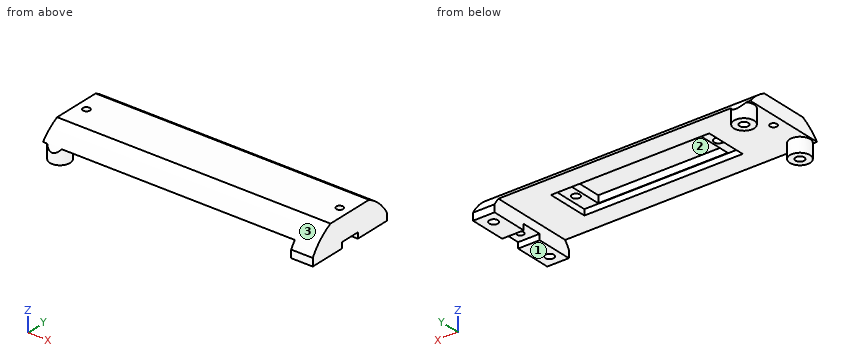
from build123d import *

# Parameters (mm, degrees)
SKETCH1_R             = 4
SKETCH1_R_2           = 1.5
BOSS_EXTRUDE1_DEPTH   = 5
BOSS_EXTRUDE1_2_DEPTH = 5
BOSS_EXTRUDE1_3_DEPTH = 5
BOSS_EXTRUDE1_4_DEPTH = 5
SKETCH2_W             = 95
SKETCH2_H             = 32.5
BOSS_EXTRUDE2_DEPTH   = 10
SKETCH3_W             = 45
SKETCH3_H             = 14.2
CUT_EXTRUDE1_DEPTH    = 9
SKETCH4_W             = 5
SKETCH4_H             = 14.2
SKETCH4_W_2           = 45
CUT_EXTRUDE2_DEPTH    = 4
SKETCH5_R             = 1.4
SKETCH5_R_2           = 1.6
CUT_EXTRUDE3_DEPTH    = 5
BOSS_EXTRUDE3_DEPTH   = 5
CUT_EXTRUDE5_DEPTH    = 96
SKETCH9_W             = 7
SKETCH9_H             = 7
CUT_EXTRUDE6_DEPTH    = 96
SKETCH10_R            = 1.2
CUT_EXTRUDE7_DEPTH    = 16
SKETCH12_R            = 1.5
CUT_EXTRUDE9_DEPTH    = 10
SKETCH13_W            = 95
SKETCH13_H            = 32.5
CUT_EXTRUDE10_DEPTH   = 5
SKETCH14_R            = 3.5
CUT_EXTRUDE11_DEPTH   = 5
SKETCH15_W            = 45
SKETCH15_H            = 14.2
CUT_EXTRUDE12_DEPTH   = 0.5
SKETCH16_R            = 1.4
SKETCH16_R_2          = 1.6
SKETCH16_W            = 45
SKETCH16_H            = 14.2
CUT_EXTRUDE13_DEPTH   = 2


with BuildPart() as part:
    # Sketch1 → Boss-Extrude1 (new body)
    with BuildSketch(Plane.XY):
        with Locations((-43.5, -12.25)):
            Circle(SKETCH1_R)
        with Locations((-43.5, -12.25)):
            Circle(SKETCH1_R_2, mode=Mode.SUBTRACT)
    extrude(amount=BOSS_EXTRUDE1_DEPTH)



with BuildPart() as body_2:
    # Sketch1 → Boss-Extrude1 2 (new body)
    with BuildSketch(Plane.XY):
        with Locations((-43.5, 12.25)):
            Circle(SKETCH1_R)
        with Locations((-43.5, 12.25)):
            Circle(SKETCH1_R_2, mode=Mode.SUBTRACT)
    extrude(amount=BOSS_EXTRUDE1_2_DEPTH)


with BuildPart() as body_3:
    # Sketch1 → Boss-Extrude1 3 (new body)
    with BuildSketch(Plane.XY):
        with Locations((43.5, -12.25)):
            Circle(SKETCH1_R)
        with Locations((43.5, -12.25)):
            Circle(SKETCH1_R_2, mode=Mode.SUBTRACT)
    extrude(amount=BOSS_EXTRUDE1_3_DEPTH)


with BuildPart() as body_4:
    # Sketch1 → Boss-Extrude1 4 (new body)
    with BuildSketch(Plane.XY):
        with Locations((43.5, 12.25)):
            Circle(SKETCH1_R)
        with Locations((43.5, 12.25)):
            Circle(SKETCH1_R_2, mode=Mode.SUBTRACT)
    extrude(amount=BOSS_EXTRUDE1_4_DEPTH)


with BuildPart() as part_1:
    add(part.part)

    add(body_2.part)  # Boss-Extrude2 merges body 2

    add(body_3.part)  # Boss-Extrude2 merges body 3

    add(body_4.part)  # Boss-Extrude2 merges body 4
    # Sketch2 → Boss-Extrude2 (add)
    with BuildSketch(Plane.XY.offset(5)):
        Rectangle(SKETCH2_W, SKETCH2_H)
    extrude(amount=BOSS_EXTRUDE2_DEPTH)

    # Sketch3 → Cut-Extrude1 (cut)
    with BuildSketch(Plane(origin=(0, 0, 5), x_dir=(-1, 0, 0), z_dir=(0, 0, -1))):
        Rectangle(SKETCH3_W, SKETCH3_H)
    extrude(amount=-CUT_EXTRUDE1_DEPTH, mode=Mode.SUBTRACT)

    # Sketch4 → Cut-Extrude2 (cut)
    with BuildSketch(Plane(origin=(0, 0, 5), x_dir=(-1, 0, 0), z_dir=(0, 0, -1))):
        with Locations((-25, 0)):
            Rectangle(SKETCH4_W, SKETCH4_H)
        Rectangle(SKETCH4_W_2, SKETCH4_H)
        with Locations((25, 0)):
            Rectangle(SKETCH4_W, SKETCH4_H)
    extrude(amount=-CUT_EXTRUDE2_DEPTH, mode=Mode.SUBTRACT)

    # Sketch5 → Cut-Extrude3 (cut)
    with BuildSketch(Plane(origin=(0, 0, 9), x_dir=(-1, 0, 0), z_dir=(0, 0, -1))):
        with Locations((-24.8, -0.2)):
            Circle(SKETCH5_R)
        with Locations((24.8, -0.2)):
            Circle(SKETCH5_R_2)
    extrude(amount=-CUT_EXTRUDE3_DEPTH, mode=Mode.SUBTRACT)

    # Sketch6 → Boss-Extrude3 (add)
    with BuildSketch(Plane(origin=(0, 0, 5), x_dir=(-1, 0, 0), z_dir=(0, 0, -1))):
        with BuildLine():
            ThreePointArc((47.5, 12.25), (43.5, 8.25), (39.5, 12.25))
            Line((39.5, 12.25), (39.5, -12.25))
            ThreePointArc((39.5, -12.25), (43.5, -8.25), (47.5, -12.25))
            Line((47.5, -12.25), (47.5, 12.25))
        make_face()
        with BuildLine():
            ThreePointArc((-39.5, 12.25), (-43.5, 8.25), (-47.5, 12.25))
            Line((-47.5, 12.25), (-47.5, -12.25))
            ThreePointArc((-47.5, -12.25), (-43.5, -8.25), (-39.5, -12.25))
            Line((-39.5, -12.25), (-39.5, 12.25))
        make_face()
    extrude(amount=BOSS_EXTRUDE3_DEPTH)

    # Sketch8 → Cut-Extrude5 (cut, through all)
    with BuildSketch(Plane(origin=(47.5, 0, 0), x_dir=(0, 0, -1), z_dir=(1, 0, 0))):
        with BuildLine():
            ThreePointArc((-15, 8.377014021), (-11.841659381, 12.867099577), (-7.518238456, 16.25))
            Line((-7.518238456, 16.25), (-15, 16.25))
            Line((-15, 16.25), (-15, 8.377014021))
        make_face()
        with BuildLine():
            Line((-15, -16.25), (-7.688934819, -16.25))
            ThreePointArc((-7.688934819, -16.25), (-11.909309532, -12.893789895), (-15, -8.475267356))
            Line((-15, -8.475267356), (-15, -16.25))
        make_face()
    extrude(amount=-CUT_EXTRUDE5_DEPTH, mode=Mode.SUBTRACT)

    # Sketch9 → Cut-Extrude6 (cut, through all)
    with BuildSketch(Plane.ZY.offset(47.5)):
        with Locations((3.5, 0)):
            Rectangle(SKETCH9_W, SKETCH9_H)
    extrude(amount=-CUT_EXTRUDE6_DEPTH, mode=Mode.SUBTRACT)

    # Sketch10 → Cut-Extrude7 (cut, through all)
    with BuildSketch(Plane.XY.offset(15)):
        with Locations((-44, -0.049126667)):
            Circle(SKETCH10_R)
        with Locations((44, -0.049126667)):
            Circle(SKETCH10_R)
    extrude(amount=-CUT_EXTRUDE7_DEPTH, mode=Mode.SUBTRACT)

    # Sketch12 → Cut-Extrude9 (cut)
    with BuildSketch(Plane(origin=(0, 0, 0), x_dir=(-1, 0, 0), z_dir=(0, 0, -1))):
        with Locations((-43.5, 12.25)):
            Circle(SKETCH12_R)
        with Locations((-43.5, -12.25)):
            Circle(SKETCH12_R)
        with Locations((43.5, 12.25)):
            Circle(SKETCH12_R)
        with Locations((43.5, -12.25)):
            Circle(SKETCH12_R)
    extrude(amount=-CUT_EXTRUDE9_DEPTH, mode=Mode.SUBTRACT)

    # Sketch13 → Cut-Extrude10 (cut)
    with BuildSketch(Plane(origin=(0, 0, 0), x_dir=(-1, 0, 0), z_dir=(0, 0, -1))):
        Rectangle(SKETCH13_W, SKETCH13_H)
    extrude(amount=-CUT_EXTRUDE10_DEPTH, mode=Mode.SUBTRACT)

    # Sketch14 → Cut-Extrude11 (cut)
    with BuildSketch(Plane(origin=(0, 0, 5), x_dir=(-1, 0, 0), z_dir=(0, 0, -1))):
        Polygon((-40, 16.25), (-40, -3.5), (-27.5, -3.5), (-27.5, -7.1), (27.5, -7.1), (27.5, -3.5), (47.5, -3.5), (47.5, 16.25), align=None)
        with Locations((43.5, 12.25)):
            Circle(SKETCH14_R, mode=Mode.SUBTRACT)
        Polygon((-40, -3.5), (-40, -12.25), (-40, -16.25), (47.5, -16.25), (47.5, -3.5), (27.5, -3.5), (27.5, -7.1), (-27.5, -7.1), (-27.5, -3.5), align=None)
        with Locations((43.5, -12.25)):
            Circle(SKETCH14_R, mode=Mode.SUBTRACT)
    extrude(amount=-CUT_EXTRUDE11_DEPTH, mode=Mode.SUBTRACT)

    # Sketch15 → Cut-Extrude12 (cut)
    with BuildSketch(Plane(origin=(0, 0, 14), x_dir=(-1, 0, 0), z_dir=(0, 0, -1))):
        Rectangle(SKETCH15_W, SKETCH15_H)
    extrude(amount=-CUT_EXTRUDE12_DEPTH, mode=Mode.SUBTRACT)

    # Sketch16 → Cut-Extrude13 (cut)
    with BuildSketch(Plane(origin=(0, 0, 10), x_dir=(-1, 0, 0), z_dir=(0, 0, -1))):
        Polygon((-27.5, 7.3), (-27.5, 7.1), (-27.5, -7.3), (27.5, -7.3), (27.5, -7.1), (27.5, 7.3), align=None)
        with Locations((-24.8, -0.2)):
            Circle(SKETCH16_R, mode=Mode.SUBTRACT)
        with Locations((24.8, -0.2)):
            Circle(SKETCH16_R_2, mode=Mode.SUBTRACT)
        Rectangle(SKETCH16_W, SKETCH16_H, mode=Mode.SUBTRACT)
        Rectangle(SKETCH16_W, SKETCH16_H)
    extrude(amount=-CUT_EXTRUDE13_DEPTH, mode=Mode.SUBTRACT)


solid = part_1.part
Design review of the part built by this model. Coordinates are the model's own, in mm. Face numbers are marked on the shaded views. Coordinates: 2 decimals unless noted, no trailing zeros. Order: outer loops, then holes, each group sorted by start corner. A loop starts at its lowest first (then second) coordinate and runs counter-clockwise, first axis right, second up.
Item 1: Take a section at A-A, the plane x = 2. Write out the cut boundary in (y, z).
Item 2: For line 1 (X direction, y = -12.25, z = 7.3); line 2 (Y direction, x = -43.5, z = 7.4); line 3 (Z direction, x = -35, y = -1.5), list the stretches that pass through material, from the lowest coordinate up.
Item 3: Take a section at B-B, the plane x = 44. Write out the cut boundary in (y, z).
Item 4: The part is to be moulded in two halves that separate along Y. For the marked faces 1, 2 and 3, say which applies: pulls with the +Y half, pulls with the -Y half, needs draft (parallel to the pull), parting line crosses it, or undercut.
Item 5: For pin 1 Ø2.5 at (x, y) = (43.5, 12.25) entering from -Z; pin 2 Ø3 at (x, y) = (24.5, 0) entering from -Z; pin 3 Ø2.5 at (x, y) = (-43.5, -12.25) entering from +Z, all flat-tipped, find the tip position at first contact; note any pin that passes through.
Item 6: Take a section at D-D, the plane x = 32. Write out the cut boundary in (y, z).
Item 7: Take a section at C-C, the plane y = -12.25. Write out the cut boundary in (x, z).
The answers:
1. outline: (-14.66, 10) - (-7.3, 10) - (-7.3, 12) - (-7.1, 12) - (-7.1, 14.5) - (7.1, 14.5) - (7.1, 12) - (7.3, 12) - (7.3, 10) - (14.56, 10) arc R18.75 ccw to (8.38, 15) - (-8.48, 15) arc R18.75 ccw to start
2. line 1: x = -47 to -45, -42 to -40, 40 to 42, 45 to 47.5
2. line 2: y = -15.75 to -13.75, -10.75 to -8.75, 8.75 to 10.75, 13.75 to 15.75
2. line 3: z = 10 to 15
3. outline: (-16.25, 5) - (-13.66, 5) - (-13.66, 10) - (-10.84, 10) - (-10.84, 5) - (-3.5, 5) - (-3.5, 7) - (-1.25, 7) - (-1.25, 15) - (-8.48, 15) arc R18.75 ccw to (-16.25, 7.69) - close; (1.15, 7) - (3.5, 7) - (3.5, 5) - (10.84, 5) - (10.84, 10) - (13.66, 10) - (13.66, 5) - (16.25, 5) - (16.25, 7.52) arc R18.75 ccw to (8.38, 15) - (1.15, 15) - close
4. face 1: needs draft
4. face 2: undercut
4. face 3: pulls with the -Y half
5. pin 1: stops at z = 10
5. pin 2: stops at z = 12
5. pin 3: stops at z = 13.47
6. outline: (-14.66, 10) - (14.56, 10) arc R18.75 ccw to (8.38, 15) - (-8.48, 15) arc R18.75 ccw to start
7. outline: (-47.5, 10) - (-47, 10) - (-47, 5) - (-45, 5) - (-45, 10) - (-42, 10) - (-42, 5) - (-40, 5) - (-40, 10) - (40, 10) - (40, 5) - (42, 5) - (42, 10) - (45, 10) - (45, 5) - (47.5, 5) - (47.5, 12.49) - (-47.5, 12.49) - close
